Part model, mm, in its own coordinate system. A direction names the side the tool comes from. Round coordinates to 2 decimals unless told otherwise and drop trailing zeros. Order: outer loops, then holes, each group sorted by start corner. A loop starts at its lowest first (then second) coordinate and runs counter-clockwise, first axis right, second up. Notation, with made-up numbers: (69, 48.25) - (107, 48.25) arc R18 cw to (107, 65.25) - close; hole circle Ø2 at (-11, 15). An arc over 180 degrees is marked (long way). Return JSON: item names as keys, results as strings. Group by question number.
Item 1: Tool access for faces 4 (the face through (232, -12.7, 0)), 5 (the face through (232, 0, 3.175)): list every direction of +Z, -Z, +X, -X, +Y, -Y with a clear straight run to the whole face (end or side of a thin tool).
Item 2: Saw through at B-B on x = 138. List the corners of the cut face in (y, z) (3 decimals), and give its area (3 significant figures).
Item 3: Two-plate mould, pull along Z, no slides. Class faces 1 (the face through (232, 0, 6.35)), 2 (the face through (469.9, 0, 4)), 3 (the face through (232, 0, -3.175)): released by +Z, released by -Z, zero draft, split by the parting line, or undercut.
Item 4: Probe probe 1 along Z at (x, y) = (288.5, 7.25) (3 decimals); probe 2 along X at (y, z) = (6.35, -5.5); probe 3 along Y at (x, z) = (45.5, -1.5) (3 decimals). List the from-to ranges inside material, lowest first.
Item 5: Saw through at A-A on z = -1. List the corners of the cut face in (x, y) (3 decimals).
Item 6: Drop a flat-ended pin along its axis: pin 1 (5 mm diameter, centred on x = 319.82, y = 0, fed in from +Z) (3 decimals). Give the stop position or say it passes through.
```python
from build123d import *

# Parameters (mm, degrees)
F0_W     = 25.4
F0_H     = 12.7
F0_W_2   = 19.05
F0_H_2   = 6.35
F1_DEPTH = 469.9
F4_D     = 2.7051
F4_DEPTH = 3.175
F4_TIP   = 0.8126940303
F5_R     = 3.175
F6_DEPTH = 3.175


with BuildPart() as f1:
    # F0 (on Right) → F1 (new body)
    with BuildSketch(Plane.YZ):
        Rectangle(F0_W, F0_H)
        Rectangle(F0_W_2, F0_H_2, mode=Mode.SUBTRACT)
    extrude(amount=F1_DEPTH)

    # F4
    with Locations(Plane(origin=(0, 0, -6.35), x_dir=(1, 0, 0), z_dir=(0, 0, -1))):
        with Locations((16.002, -6.35), (16.002, 6.35), (66.802, 6.35), (66.802, -6.35)):
            Hole(F4_D / 2, depth=F4_DEPTH)
            with Locations((0, 0, -(F4_DEPTH + F4_TIP / 2))):  # 118° drill point
                Cone(0, F4_D / 2, F4_TIP, mode=Mode.SUBTRACT)

    # F5 (on face) → F6 (cut)
    with BuildSketch(Plane.XY.offset(6.35)):
        with Locations((380.994543826, 6.90038e-05)):
            Circle(F5_R)
        with Locations((319.818643826, 6.90038e-05)):
            Circle(F5_R)
        with Locations((265.310243826, 6.90038e-05)):
            Circle(F5_R)
        with Locations((216.745443826, 6.90038e-05)):
            Circle(F5_R)
        with BuildLine():
            Line((150.476843826, 3.8100690038), (150.476843826, -3.8099309962))
            ThreePointArc((150.476843826, -3.8099309962), (153.651843826, -6.9849309962), (156.826843826, -3.8099309962))
            Line((156.826843826, -3.8099309962), (156.826843826, 3.8100690038))
            ThreePointArc((156.826843826, 3.8100690038), (153.651843826, 6.9850690038), (150.476843826, 3.8100690038))
        make_face()
        with Locations((100.591243826, 6.90038e-05)):
            Circle(F5_R)
        with Locations((69.984243826, 6.90038e-05)):
            Circle(F5_R)
        with Locations((42.730043826, 6.90038e-05)):
            Circle(F5_R)
        with Locations((18.434943826, 6.90038e-05)):
            Circle(F5_R)
    extrude(amount=-F6_DEPTH, mode=Mode.SUBTRACT)


solid = f1.part
```
Filled in:
{
 "1": {"face 4": "+Z, -Z, +X, -X, -Y", "face 5": "+X, -X"},
 "2": {"outline": "(-12.7, -6.35) - (12.7, -6.35) - (12.7, 6.35) - (-12.7, 6.35) - close; hole (-9.525, -3.175) - (9.525, -3.175) - (9.525, 3.175) - (-9.525, 3.175) - close", "area": "202 mm^2"},
 "3": {"face 1": "released by +Z", "face 2": "zero draft", "face 3": "undercut"},
 "4": {"probe 1": "z = -6.35 to -3.175, 3.175 to 6.35", "probe 2": "x = 0 to 14.65, 17.35 to 65.45, 68.15 to 469.9", "probe 3": "y = -12.7 to -9.525, 9.525 to 12.7"},
 "5": {"outline": "(0, -12.7) - (469.9, -12.7) - (469.9, -9.525) - (0, -9.525) - close; (0, 9.525) - (469.9, 9.525) - (469.9, 12.7) - (0, 12.7) - close"},
 "6": {"pin 1": "stops at z = -3.175"}
}
